Source: CAD feature listing. Evaluate the final solid. Frame: model axes, mm. A direction names the side the tool comes from. Round coordinates to 2 decimals unless told otherwise and drop trailing zeros. Order: outer loops, then holes, each group sorted by start corner. A loop starts at its lowest first (then second) coordinate and runs counter-clockwise, first axis right, second up. Notation, with made-up numbers: (69.25, 74.25) -> (109.25, 74.25) arc R12 ccw to (109.25, 87.25) -> close; hole circle Ø10 at (8.25, 80). An arc over 180 degrees is marked (long way). One line per item, written item: value. Start each with the question number.
1) Mould query, pull axis Y, two halves, no side actions, for faces 3 (the face through (6, 2, 8)), 4 (the face through (-6, 50, 600)), 5 (the face through (-2.136, 50.268, 500.986)). Classes: pulls with the +Y half, pulls with the -Y half, needs draft (parallel to the pull), parting line crosses it, or undercut.
2) Section C-C (z = -1.5). Return the cut outline in (x, y), and give its area (3 significant figures).
3) Reachability of faces 1 (the face through (6, 0, 8)), 2 (the face through (-350, 194, -7)) from +Z, -Z, +X, -X, +Y, -Y: full face, straight path, thin tool, end or side. Return the list, or none.
4) Section B-B (x = -310). Return the cut outline in (y, z), and give its area (3 significant figures).
5) Ray query, L1, parallel to Z at x = -119, y = 47; L2, parallel to Z at x = -392, y = 1; L3, parallel to X at y = 32, z = 359.5. Return the intervals inside material, ascending.
6) Section A-A (y = 172). Return the cut outline in (x, z), and give its area (3 significant figures).
7) Section D-D (y = 62). State how many separate pieces and enclosed holes the cut face has, and give its area (3 significant figures).
8) Pin query (flat end, axial travel): P1, Ø3, axis at x = 279.5, z = 329, coming from the -Y side; P2, Ø1.5, axis at y = 171, z = -260.5, coming from the +X side; P3, Ø1.5, axis at x = -339, y = 253.5, coming from the -Z side; P4, Ø12, axis at x = -392, z = 197, coming from the +Y side. Return the tip coordinate at first contact, or that it passes through.
Autodesk Inventor part; units mm, degrees
ref_plane "YZ Plane" through (0, 0, 0) normal (1, 0, 0) x (0, 1, 0)
ref_plane "XZ Plane" through (0, 0, 0) normal (0, 1, 0) x (-1, 0, 0)
ref_plane "XY Plane" through (0, 0, 0) normal (0, 0, 1) x (1, 0, 0)
sketch "Sketch1" plane through (0, 0, 0) normal (0, 1, 0) x (-1, 0, 0)
  line L0 (345, 500) -> (-345, 500)
  line L1 (-345, -500) -> (345, -500)
  line L2 (350, -495) -> (350, 495)
  line L3 (350, 500) -> (-350, -500) construction
  line L4 (-350, 500) -> (350, -500) construction
  line L5 (347, 502) -> (-347, 502)
  line L6 (-347, -502) -> (347, -502)
  line L7 (352, -497) -> (352, 497)
  line L8 (352, 502) -> (-352, -502) construction
  line L9 (-352, 502) -> (352, -502) construction
  line L10 (445, 600) -> (-445, 600)
  line L11 (-450, 595) -> (-450, -595)
  line L12 (-445, -600) -> (445, -600)
  line L13 (450, -595) -> (450, 595)
  line L14 (450, 600) -> (-450, -600) construction
  line L15 (-450, 600) -> (450, -600) construction
  line L16 (447, 602) -> (-447, 602)
  line L17 (-452, 597) -> (-452, -597)
  line L18 (-447, -602) -> (447, -602)
  line L19 (452, -597) -> (452, 597)
  line L20 (452, 602) -> (-452, -602) construction
  line L21 (-452, 602) -> (452, -602) construction
  arc A0 (452, 597) -> (447, 602) centre (447, 597) ccw
  arc A1 (450, 595) -> (445, 600) centre (445, 595) ccw
  arc A2 (-445, 600) -> (-450, 595) centre (-445, 595) ccw
  arc A3 (-447, 602) -> (-452, 597) centre (-447, 597) ccw
  arc A4 (-450, -595) -> (-445, -600) centre (-445, -595) ccw
  arc A5 (-452, -597) -> (-447, -602) centre (-447, -597) ccw
  arc A6 (445, -600) -> (450, -595) centre (445, -595) ccw
  arc A7 (447, -602) -> (452, -597) centre (447, -597) ccw
  arc A8 (350, 495) -> (345, 500) centre (345, 495) ccw
  arc A9 (352, 497) -> (347, 502) centre (347, 497) ccw
  arc A10 (-345, 500) -> (-350, 495) centre (-345, 495) ccw
  arc A11 (-347, 502) -> (-352, 497) centre (-347, 497) ccw
  arc A12 (-352, -497) -> (-347, -502) centre (-347, -497) ccw
  arc A13 (-350, -495) -> (-345, -500) centre (-345, -495) ccw
  arc A14 (345, -500) -> (350, -495) centre (345, -495) ccw
  arc A15 (347, -502) -> (352, -497) centre (347, -497) ccw
  line L22 (-350, 495) -> (-352, 495)
  line L23 (-350, -495) -> (-352, -495)
  line L24 (-352, 497) -> (-352, 495)
  line L25 (-350, 466.6667) -> (-350, 466.1504)
  line L26 (-352, 469.3333) -> (-352, 468.8142)
  line L27 (-352, -495) -> (-352, -497)
  point P0 (0, 0)
  dimension "d0" = 700
  dimension "d1" = 1000
  dimension "d2" = 704
  dimension "d3" = 1004
  dimension "d4" = 900
  dimension "d5" = 1200
  dimension "d6" = 904
  dimension "d7" = 1204
  dimension "d8" = 5
  dimension "d9" = 5
extrude "Extrusion6" add sketch "Sketch1" along normal blind 2 contours A1 L13 A6 L12 A4 L11 A2 L10
extrude "Extrusion7" add sketch "Sketch1" along normal blind 392 contours L0 A10 L22 L24 A11 L5 A9 L7 A15 L6 A12 L27 L23 A13 L1 A14 L2 A8
extrude "Extrusion8" add sketch "Sketch1" along normal blind 100 contours A0 L19 A7 L18 A5 L17 A3 L16
sketch "Sketch2" plane through (-347, 2, 502) normal (0, 0, 1) x (1, 0, 0)
  line L0 (694, 0) -> (694, 390)
  line L1 (0, 390) -> (694, 390)
  point P0 (347, -2)
  point P1 (347, 200)
  dimension "d40" = 347
  dimension "d42" = 190
hole "Hole1" at (0, 202, 502) direction (0, 0, -1) diameter 5 depth 3 tip angle 118
sketch "Sketch3" plane through (-347, 2, 502) normal (0, 0, 1) x (1, 0, 0)
  line L0 (694, 0) -> (694, 390)
  line L1 (0, 390) -> (694, 390)
  point P0 (347, -2)
  point P1 (347, 170)
  dimension "d41" = 347
  dimension "d43" = 220
hole "Hole2" at (0, 172, 502) direction (0, 0, -1) diameter 30 depth 3 tip angle 118
sketch "Sketch4" plane through (-352, 2, 497) normal (-1, 0, 0) x (0, 0, 1)
  line L0 (0, 0) -> (0, 390)
  line L1 (-994, 390) -> (0, 390)
  point P0 (-497, -2)
  point P1 (-150, -20)
  point P2 (-300, 310)
  dimension "d58" = 300
  dimension "d59" = 150
  dimension "d60" = 80
  dimension "d61" = 410
hole "Hole3" at (-352, -18, 347) at (-352, 312, 197) direction (1, 0, 0) diameter 20 depth 20
sketch "Sketch5" plane through (0, 2, 0) normal (0, 1, 0) x (1, 0, 0)
  line L0 (-352, -497) -> (-352, 497)
  point P0 (0, 0)
  point P1 (-392, -347)
  point P2 (-392, -197)
  dimension "d62" = 150
  dimension "d63" = 40
  dimension "d64" = 300
  dimension "d65" = 40
hole "Hole4" at (-392, 2, 347) at (-392, 2, 197) direction (0, -1, 0) diameter 20 depth 20
sketch "Sketch6" plane through (-347, 2, 502) normal (0, 0, 1) x (1, 0, 0)
  line L0 (694, 0) -> (0, 0)
  line L1 (0, 0) -> (0, 390)
  point P0 (347, -2)
  point P1 (340, 60)
  dimension "d73" = 60
  dimension "d74" = 340
hole "Hole5" at (-7, 62, 502) direction (0, 0, -1) diameter 25.4 depth 25.4 tip angle 118
sketch "Sketch7" plane through (0, 2, 0) normal (0, 1, 0) x (1, 0, 0)
  point P0 (0, 0)
  point P1 (-5, -535.191)
  point P2 (-345, -500)
  dimension "d82" = 340
hole "Hole6" at (-5, 2, 535.191) direction (0, -1, 0) diameter 26 depth 26 tip angle 118
properties part number "tub" material "CFRP"
Findings:
1. face 3: pulls with the +Y half
1. face 4: needs draft
1. face 5: undercut
2. outline: (-452, 0) -> (452, 0) -> (452, 100) -> (450, 100) -> (450, 2) -> (-350, 2) -> (-350, 392) -> (-352, 392) -> (-352, 2) -> (-450, 2) -> (-450, 100) -> (-452, 100) -> close
2. area: 2,980 mm2
3. face 1: +Z, -Z, +X, -X, -Y
3. face 2: +Y
4. outline: (0, -602) -> (100, -602) -> (100, -600) -> (2, -600) -> (2, -502) -> (392, -502) -> (392, -500) -> (2, -500) -> (2, 500) -> (392, 500) -> (392, 502) -> (2, 502) -> (2, 600) -> (100, 600) -> (100, 602) -> (0, 602) -> close
4. area: 4,360 mm2
5. L1: -602 to -600, -502 to -500, 500 to 502, 600 to 602
5. L2: -602 to 187, 207 to 337, 357 to 602
5. L3: -452 to -450, -352 to -350, 450 to 452
6. outline: (-352, -497) arc R5 ccw to (-347, -502) -> (347, -502) arc R5 ccw to (352, -497) -> (352, -495) -> (350, -495) arc R5 cw to (345, -500) -> (-345, -500) arc R5 cw to (-350, -495) -> (-350, 495) arc R5 cw to (-345, 500) -> (-15, 500) -> (-15, 502) -> (-347, 502) arc R5 ccw to (-352, 497) -> close; (15, 500) -> (345, 500) arc R5 cw to (350, 495) -> (352, 495) -> (352, 497) arc R5 ccw to (347, 502) -> (15, 502) -> close
6. area: 4,780 mm2
7. separate pieces: 3
7. enclosed holes: 1
7. area: 13,200 mm2
8. P1: y = 0
8. P2: x = -350
8. P3: z = -502
8. P4: through
